Geometry: final body of the model. Coordinates: model frame, mm. A direction names the side the tool comes from. Round coordinates to 2 decimals unless told otherwise and drop trailing zeros. Loops run counter-clockwise (first coordinate to the right, second up) from the corner with the lowest first, then second, coordinate; pieces in that order, holes last. Notation, with made-up numbers: (-35, 68.5) -> (-8, 68.5) arc R31 ccw to (-8, 92.5) -> close; hole circle Ø7 at (28.25, -18.5). An arc over 180 degrees is marked (long way). Answer in a Markdown table with one row per item.
```python
from build123d import *

# Parameters (mm, degrees)
SKETCH1_R           = 15
BOSS_EXTRUDE1_DEPTH = 20
BOSS_EXTRUDE2_DEPTH = 10
SKETCH3_R           = 0.75
BOSS_EXTRUDE3_DEPTH = 3


with BuildPart() as part:
    # Sketch1 → Boss-Extrude1 (new body)
    with BuildSketch(Plane.XY):
        Circle(SKETCH1_R)
    extrude(amount=BOSS_EXTRUDE1_DEPTH)

    # Sketch2 → Boss-Extrude2 (add)
    with BuildSketch(Plane.XY.offset(20)):
        with BuildLine():
            Line((-6.495190528, -3.75), (-10.825317547, -6.25))
            ThreePointArc((-10.825317547, -6.25), (0, 12.5), (10.825317547, -6.25))
            Line((10.825317547, -6.25), (6.495190528, -3.75))
            ThreePointArc((6.495190528, -3.75), (0, 7.5), (-6.495190528, -3.75))
        make_face()
    extrude(amount=BOSS_EXTRUDE2_DEPTH)

    # Sketch3 → Boss-Extrude3 (add)
    with BuildSketch(Plane.XY.offset(30)):
        with Locations((9.5, 0)):
            Circle(SKETCH3_R)
        with Locations((-9.5, 0)):
            Circle(SKETCH3_R)
    extrude(amount=BOSS_EXTRUDE3_DEPTH)


solid = part.part
```
Item 1: Draft query along X for faces 4 (the face through (8.691, -5.018, 24.93)), 5 (the face through (9, 0, 33)), 6 (the face through (-14.985, 0.66, 9.86)). Return one class per face: pulls with the +X half, pulls with the -X half, needs draft (parallel to the pull), parting line crosses it, or undercut.
Answer:
| item | result |
|---|---|
| face 4 | undercut |
| face 5 | needs draft |
| face 6 | parting line crosses it |
Item 2: Pin query (flat end, axial travel): pin 1 Ø1.5 at (x, z) = (-2, 28.5) entering from +Y; pin 2 Ø5 at (x, z) = (7, 5.5) entering from -Y; pin 3 Ø8 at (y, z) = (-10.5, 10.5) entering from -X. Return the tip coordinate at first contact, or that it passes through.
Answer:
| item | result |
|---|---|
| pin 1 | stops at y = 12.44 |
| pin 2 | stops at y = -14.31 |
| pin 3 | stops at x = -13.52 |
Item 3: Line query: probe 1 along X at (y, z) = (0, 23.25); probe 2 along Z at (x, y) = (5.5, -7); probe 3 along Y at (x, z) = (0, 28.25). Output: solid intervals per line, ascending. Write a range as [from, to].
Answer:
| item | result |
|---|---|
| probe 1 | x = [-12.5, -7.5], [7.5, 12.5] |
| probe 2 | z = [0, 20] |
| probe 3 | y = [7.5, 12.5] |
Item 4: Reachability of faces 1 (the face through (0, -3, 20)), 2 (the face through (-8.63, -4.983, 24.93)), 3 (the face through (-10, 0, 33)) from +Z, -Z, +X, -X, +Y, -Y: full face, straight path, thin tool, end or side. Return the list, or none.
Answer:
| item | result |
|---|---|
| face 1 | +Z |
| face 2 | +Z, -Y |
| face 3 | +Z, +X, -X, +Y, -Y |
Item 5: Cut plane C-C (z = 21). Output: boundary loops of the cut face in (x, y).
Answer:
| item | result |
|---|---|
| outline | (-10.83, -6.25) -> (-6.5, -3.75) arc R7.5 cw (long way) to (6.5, -3.75) -> (10.83, -6.25) arc R12.5 ccw (long way) to start |
Item 6: Cut plane B-B (y = 0). Output: boundary loops of the cut face in (x, z).
Answer:
| item | result |
|---|---|
| outline | (-15, 0) -> (15, 0) -> (15, 20) -> (12.5, 20) -> (12.5, 30) -> (10.25, 30) -> (10.25, 33) -> (8.75, 33) -> (8.75, 30) -> (7.5, 30) -> (7.5, 20) -> (-7.5, 20) -> (-7.5, 30) -> (-8.75, 30) -> (-8.75, 33) -> (-10.25, 33) -> (-10.25, 30) -> (-12.5, 30) -> (-12.5, 20) -> (-15, 20) -> close |
Item 7: Cut plane A-A (x = 0). Output: boundary loops of the cut face in (y, z), then the cut area to 3 significant figures.
Answer:
| item | result |
|---|---|
| outline | (-15, 0) -> (15, 0) -> (15, 20) -> (12.5, 20) -> (12.5, 30) -> (7.5, 30) -> (7.5, 20) -> (-15, 20) -> close |
| area | 650 mm² |
Item 8: Cut plane D-D (x = 9.5). Output: boundary loops of the cut face in (y, z).
Answer:
| item | result |
|---|---|
| outline | (-11.61, 0) -> (11.61, 0) -> (11.61, 20) -> (8.12, 20) -> (8.12, 30) -> (0.75, 30) -> (0.75, 33) -> (-0.75, 33) -> (-0.75, 30) -> (-5.48, 30) -> (-5.48, 20) -> (-11.61, 20) -> close |
